```python
from build123d import *

# Parameters (mm, degrees)
SKETCH3_W           = 330.2
SKETCH3_H           = 6.35
BOSS_EXTRUDE1_DEPTH = 511.175
SKETCH4_R           = 8.128
CUT_EXTRUDE1_DEPTH  = 7.35


with BuildPart() as part:
    # Sketch3 → Boss-Extrude1 (new body)
    with BuildSketch(Plane.XY):
        with Locations((165.1, 3.175)):
            Rectangle(SKETCH3_W, SKETCH3_H)
    extrude(amount=-BOSS_EXTRUDE1_DEPTH)

    # Sketch4 → Cut-Extrude1 (cut, through all)
    with BuildSketch(Plane(origin=(0, 0, 0), x_dir=(1, 0, 0), z_dir=(0, 1, 0))):
        with Locations((101.6, 25.4)):
            Circle(SKETCH4_R)
        with Locations((225.199138423, 25.4)):
            Circle(SKETCH4_R)
        with Locations((225.199138423, 485.775)):
            Circle(SKETCH4_R)
        with Locations((101.6, 485.775)):
            Circle(SKETCH4_R)
    extrude(amount=CUT_EXTRUDE1_DEPTH, mode=Mode.SUBTRACT)


solid = part.part
```
Here's how the part is built. I have some questions about the finished solid (model axes, mm). Coordinates: 2 decimals unless noted, no trailing zeros. Order: outer loops, then holes, each group sorted by start corner. A loop starts at its lowest first (then second) coordinate and runs counter-clockwise, first axis right, second up. Notation, with made-up numbers: (76, 12) - (106, 12) arc R18 cw to (106, 47) - close; hole circle Ø3 at (23.5, 64.25). An arc over 180 degrees is marked (long way). One line per question, with ' | ' between items. Start each with the question number.
1. Please list where these lines run through material, in increasing order: line 1 along Z through (x, y) = (101.6, 2.5) (3 decimals); line 2 along X through (y, z) = (3.5, -25.4); line 3 along Z through (x, y) = (218.5, 5.5) (3 decimals). Write a range as [from, to].
2. If we mould it in two halves opening along X, with no side actions, what happens to faces 1 (the flat face through (163, 0, -252)), 2 (the cylindrical face through (109.353, 3.131, -27.841))? For each: released by +X, released by -X, zero draft, split by the parting line, or undercut.
3. If we section it at A-A (z = -25.4): Write out the boundary of the cut face in (x, y).
4. If we section it at B-B (x = 101.6): Write out the boundary of the cut face in (y, z) (3 decimals), and give its area (3 significant figures).
Model answer:
1) line 1: z = [-511.175, -493.903], [-477.647, -33.528], [-17.272, 0] | line 2: x = [0, 93.47], [109.73, 217.07], [233.33, 330.2] | line 3: z = [-511.175, -490.378], [-481.172, -30.003], [-20.797, 0]
2) face 1: zero draft | face 2: undercut
3) outline: (0, 0) - (93.47, 0) - (93.47, 6.35) - (0, 6.35) - close; (109.73, 0) - (217.07, 0) - (217.07, 6.35) - (109.73, 6.35) - close; (233.33, 0) - (330.2, 0) - (330.2, 6.35) - (233.33, 6.35) - close
4) outline: (0, -511.175) - (6.35, -511.175) - (6.35, -493.903) - (0, -493.903) - close; (0, -477.647) - (6.35, -477.647) - (6.35, -33.528) - (0, -33.528) - close; (0, -17.272) - (6.35, -17.272) - (6.35, 0) - (0, 0) - close | area: 3,040 mm²
